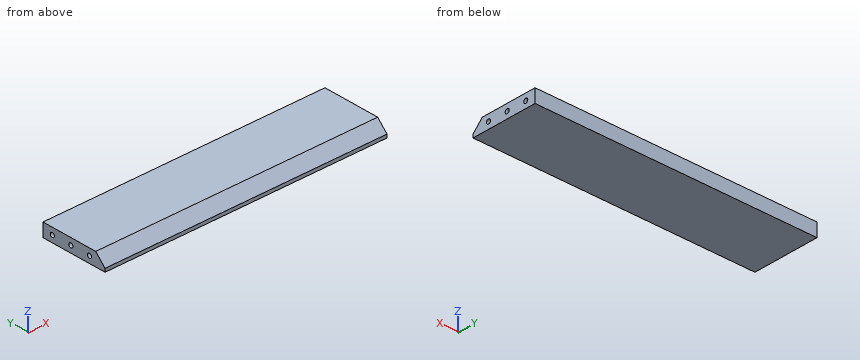
```python
from build123d import *

# Parameters (mm, degrees)
IZIM1_W                     = 420
IZIM1_H                     = 100
Y_KSEKLIK_EKSTR_ZYON1_DEPTH = 20
PAH1_SIZE                   = 15
IZIM2_R                     = 3.25
KES_EKSTR_ZYON1_DEPTH       = 30


with BuildPart() as part:
    # Çizim1 → Yükseklik-Ekstrüzyon1 (new body)
    with BuildSketch(Plane.XY):
        Rectangle(IZIM1_W, IZIM1_H)
    extrude(amount=Y_KSEKLIK_EKSTR_ZYON1_DEPTH)

    # Pah1
    pah1_edges = [part.edges().sort_by_distance(p)[0] for p in [
        (0, -50, 20),
    ]]
    chamfer(pah1_edges, length=PAH1_SIZE)

    # Çizim2 → Kes-Ekstrüzyon1 (cut)
    with BuildSketch(Plane(origin=(210, 0, 0), x_dir=(0, 0, -1), z_dir=(1, 0, 0))):
        with Locations((-10, 35)):
            Circle(IZIM2_R)
        with Locations((-10, 5)):
            Circle(IZIM2_R)
        with Locations((-10, -25)):
            Circle(IZIM2_R)
    kes_ekstr_zyon1 = extrude(amount=-KES_EKSTR_ZYON1_DEPTH, mode=Mode.SUBTRACT)

    # Aynalama1: Kes-Ekstrüzyon1 across plane
    add(kes_ekstr_zyon1.mirror(Plane(origin=(0, 0, 0), x_dir=(0, 0, 1), z_dir=(1, 0, 0))), mode=Mode.SUBTRACT)


solid = part.part
```
Here's how the part is built. I have some questions about the finished solid (model axes, mm). Give positions to 0.01 mm unless a question says otherwise; leave off trailing zeros. Write each loop counter-clockwise with the first axis right and the second up, starting at its lowest first coordinate (ties: lowest second). Pieces come first, ordered by that corner, then holes.
(1) Imagine slicing it at B-B, the plane x = -29.5. Write out the boundary of the cut face in (y, z), and give its area (3 significant figures).
Output values:
outline: (-50, 0) - (50, 0) - (50, 20) - (-35, 20) - (-50, 5) - close
area: 1,890 mm2
(2) If I drill on L1, parallel to Y at x = 192.25, z = 10; L2, parallel to Y at x = 101, z = 17.5; L3, parallel to Y at x = 10.5, z = 11.25, over which ranges is the centre line in solid material (lowest first)?
Output values:
L1: y = -45 to -28.25, -21.75 to 1.75, 8.25 to 31.75, 38.25 to 50
L2: y = -37.5 to 50
L3: y = -43.75 to 50
(3) Imagine slicing it at A-A, the plane z = 10. Write out the boundary of the cut face in (x, y), and give its area (3 significant figures).
Output values:
outline: (-210, -45) - (210, -45) - (210, -28.25) - (180, -28.25) - (180, -21.75) - (210, -21.75) - (210, 1.75) - (180, 1.75) - (180, 8.25) - (210, 8.25) - (210, 31.75) - (180, 31.75) - (180, 38.25) - (210, 38.25) - (210, 50) - (-210, 50) - (-210, 38.25) - (-180, 38.25) - (-180, 31.75) - (-210, 31.75) - (-210, 8.25) - (-180, 8.25) - (-180, 1.75) - (-210, 1.75) - (-210, -21.75) - (-180, -21.75) - (-180, -28.25) - (-210, -28.25) - close
area: 38,700 mm2
(4) Will these pins go through, and if not, where does the flat tip stop? pin 1 (10 mm diameter, centred on x = -31, y = 34.5, fed in from -Z); pin 2 (3 mm diameter, centred on y = 35.5, z = 9.5, fed in from -X); pin 3 (6 mm diameter, centred on y = -25, z = 10, fed in from +X); pin 4 (1 mm diameter, centred on x = -98, z = 14, fed in from -Y).
Output values:
pin 1: stops at z = 0
pin 2: stops at x = -180
pin 3: stops at x = 180
pin 4: stops at y = -41.5
